Here's how the part is built. I have some questions about the finished solid (model axes, mm). A direction names the side the tool comes from. Give positions to 0.01 mm unless a question says otherwise; leave off trailing zeros. Loops run counter-clockwise (first coordinate to the right, second up) from the corner with the lowest first, then second, coordinate; pieces in that order, holes last. Notation, with made-up numbers: (22, 79.25) - (62, 79.25) arc R17 ccw to (62, 108.25) - close; hole circle Ø2 at (33.25, 49). An arc over 180 degrees is marked (long way). Return JSON: item names as keys, results as strings. Group by question number.
(1) If we section it at C-C (y = 1): Please give me the cut outline in (x, z).
(2) If we section it at B-B (x = -0.5): Please give me the cut outline in (y, z).
(3) For P1, Ø2.5, axis at y = -11.5, z = 16.5, coming from the -X side; P2, Ø1.2, axis at y = -22, z = 29.5, coming from the -X side; P3, Ø4.5, axis at y = -22, z = 39, coming from the +X side, each with a flat end and sliding along its axis, tell me the tip position at first contact or that it passes through.
(4) If we section it at A-A (z = 45): Please give me the cut outline in (x, y), then the cut area to 3 significant figures.
(5) On a 3-axis mill with a long thin cutter (end or side, diameter ignored), from which of +Z, -Z, +X, -X, +Y, -Y can I reach the whole of each face in a straight line? I mean faces 1 (the flat face through (7.95, -18.52, 25.71)), 2 (the flat face through (8.04, -4.34, 20.93)), 3 (the flat face through (-5.75, -25.43, 25.71)). Say none if no direction works.
(6) If we section it at D-D (z = 16.5): Please give me the cut outline in (x, y), then the cut area to 3 significant figures.
(7) I need wall thicknesses on probe 1 along X at (y, z) = (-26.5, 42); probe 2 along X at (y, z) = (-13.5, 44.5); probe 3 along Y at (x, z) = (1, 27.5). Which ranges of each line are inside material? Lowest first, please. Write a range as [from, to].
(8) If we mould it in two halves opening along X, with no side actions, what happens to faces 4 (the flat face through (0, -24.6, 21)), 5 (the flat face through (-1.5, -27, 21)), 6 (the flat face through (0, -15, 0)), 7 (the flat face through (5, -22, 26))? For each: released by +X, released by -X, zero draft, split by the parting line, or undercut.
```python
from build123d import *

# Parameters (mm, degrees)
F1_DEPTH = 42.45
F3_W     = 13.0613458827
F3_H     = 7.237181995
F4_DEPTH = 9.7


with BuildPart() as f1:
    # F0 (on Top) → F1 (new body)
    with BuildSketch(Plane.XY):
        Polygon((5, 0), (0, 0), (0, -24.6), (1.5, -24.6), (1.5, -29.6), (6.5306729414, -29.6), (6.5306729414, -26.4880058984), (5, -24.4090993645), (5, -20.4990993645), (10.9908135316, -16.48406431), (10.9908135316, -8.5557684039), align=None)
    extrude(amount=F1_DEPTH)

    # F2: F1 across face


with BuildPart() as f1_1:
    add(f1.part)
    add(f1.part.mirror(Plane(origin=(0, -12.3, 21.225), x_dir=(0, -1, 0), z_dir=(-1, 0, 0))))

    # F3 (on face) → F4 (join)
    with BuildSketch(Plane.XY.offset(42.45)):
        Polygon((10.9908135316, -10.48406431), (14.4908135316, -10.48406431), (14.4908135316, 3.5), (-14.4908135316, 3.5), (-14.4908135316, -10.48406431), (-10.9908135316, -10.48406431), (-10.9908135316, -16.48406431), (10.9908135316, -16.48406431), align=None)
        Polygon((5, -20.4990993645), (10.9908135316, -16.48406431), (-10.9908135316, -16.48406431), (-5, -20.4990993645), (-5, -24.4090993645), (-6.5306729414, -26.4880058984), (6.5306729414, -26.4880058984), (6.3694567187, -26.2690476549), (5, -24.4090993645), align=None)
        with Locations((0, -30.106596896)):
            Rectangle(F3_W, F3_H)
    extrude(amount=F4_DEPTH)


solid = f1_1.part
```
Values:
{
 "1": {"outline": "(-14.49, 42.45) - (14.49, 42.45) - (14.49, 52.15) - (-14.49, 52.15) - close"},
 "2": {"outline": "(-33.73, 42.45) - (-24.6, 42.45) - (-24.6, 0) - (0, 0) - (0, 42.45) - (3.5, 42.45) - (3.5, 52.15) - (-33.73, 52.15) - close"},
 "3": {"P1": "x = -10.99", "P2": "x = -5", "P3": "x = 6.12"},
 "4": {"outline": "(-14.49, -10.48) - (-10.99, -10.48) - (-10.99, -16.48) - (-5, -20.5) - (-5, -24.41) - (-6.53, -26.49) - (-6.53, -33.73) - (6.53, -33.73) - (6.53, -26.49) - (5, -24.41) - (5, -20.5) - (10.99, -16.48) - (10.99, -10.48) - (14.49, -10.48) - (14.49, 3.5) - (-14.49, 3.5) - close", "area": "759 mm2"},
 "5": {"face 1": "+Z, -Z, +X", "face 2": "-Z, +X, +Y", "face 3": "+Z, -Z, -X"},
 "6": {"outline": "(-10.99, -16.48) - (-5, -20.5) - (-5, -24.41) - (-6.53, -26.49) - (-6.53, -29.6) - (-1.5, -29.6) - (-1.5, -24.6) - (1.5, -24.6) - (1.5, -29.6) - (6.53, -29.6) - (6.53, -26.49) - (5, -24.41) - (5, -20.5) - (10.99, -16.48) - (10.99, -8.56) - (5, 0) - (-5, 0) - (-10.99, -8.56) - close", "area": "464 mm2"},
 "7": {"probe 1": "[-6.53, -1.5], [1.5, 6.53]", "probe 2": "[-10.99, 10.99]", "probe 3": "[-24.6, 0]"},
 "8": {"face 4": "undercut", "face 5": "undercut", "face 6": "zero draft", "face 7": "released by +X"}
}
